Part model, mm, in its own coordinate system. A direction names the side the tool comes from. Round coordinates to 2 decimals unless told otherwise and drop trailing zeros. Write each loop counter-clockwise with the first axis right and the second up, starting at its lowest first coordinate (ties: lowest second). Pieces come first, ordered by that corner, then holes.
```python
from build123d import *

# Parameters (mm, degrees)
CHAMFER_1_SIZE           = 1
CHAMFER_2_SIZE           = 1
CHAMFER_3_SIZE           = 1
FILLET_1_R               = 2
SKETCH_2_R               = 4.5
CUT_EXTRUDE_1_DEPTH      = 72.003521039
CUT_EXTRUDE_START        = -13
SKETCH_3_R               = 7
CUT_EXTRUDE_2_DEPTH      = 9
PATTERN_CIRCULAR_2_COUNT = 4


with BuildPart() as part:
    # 草图1 → 旋转1 (revolve)
    with BuildSketch(Plane.XY, mode=Mode.PRIVATE) as revolve_1_sk:
        Polygon((45, 11), (45, 17), (23, 27.5), (23, 47.5), (10, 47.5), (10, 31), (0, 31), (0, 22.5), (15, 22.5), (15, 11), align=None)
    revolve(revolve_1_sk.sketch.rotate(Axis((0, 0, 0), (1, 0, 0)), 90), axis=Axis((0, 0, 0), (1, 0, 0)))

    # 倒角1
    chamfer_1_edges = [part.edges().sort_by_distance(p)[0] for p in [
        (45, 0, -11),
    ]]
    chamfer(chamfer_1_edges, length=CHAMFER_1_SIZE)

    # 倒角2
    chamfer_2_edges = [part.edges().sort_by_distance(p)[0] for p in [
        (0, 0, -31),
    ]]
    chamfer(chamfer_2_edges, length=CHAMFER_2_SIZE)

    # 倒角3
    chamfer_3_edges = [part.edges().sort_by_distance(p)[0] for p in [
        (23, 0, -47.5),
    ]]
    chamfer(chamfer_3_edges, length=CHAMFER_3_SIZE)

    # 圆角1
    fillet_1_edges = [part.edges().sort_by_distance(p)[0] for p in [
        (23, 0, -27.5),
    ]]
    fillet(fillet_1_edges, radius=FILLET_1_R)

    # 草图2 → 切除-拉伸1 (cut, through all)
    with BuildSketch(Plane(origin=(23, 0, 0), x_dir=(0, 0, -1), z_dir=(1, 0, 0))):
        with Locations((0, 39)):
            Circle(SKETCH_2_R)
    cut_extrude_1 = extrude(amount=-CUT_EXTRUDE_1_DEPTH, mode=Mode.SUBTRACT)

    # 草图3 → 切除-拉伸2 (cut)
    with BuildSketch(Plane.ZY.offset(-10).offset(CUT_EXTRUDE_START)):
        with Locations((0, 39)):
            Circle(SKETCH_3_R)
    cut_extrude_2 = extrude(amount=CUT_EXTRUDE_2_DEPTH, mode=Mode.SUBTRACT)

    # 阵列(圆周)2: 切除-拉伸1, 切除-拉伸2 ×4 about axis
    pattern_circular_2_axis = Axis((0, 0, 0), (1, 0, 0))
    add([cut_extrude_1.rotate(pattern_circular_2_axis, i * 360 / PATTERN_CIRCULAR_2_COUNT) for i in range(1, PATTERN_CIRCULAR_2_COUNT)], mode=Mode.SUBTRACT)
    add([cut_extrude_2.rotate(pattern_circular_2_axis, i * 360 / PATTERN_CIRCULAR_2_COUNT) for i in range(1, PATTERN_CIRCULAR_2_COUNT)], mode=Mode.SUBTRACT)


solid = part.part
```
Q1. Cut at C-C on x = 38.5. Write the cut outline in (y, z), plus the area to 3 significant figures.
Values follow:
outline: circle Ø40.2 at (0, 0); hole circle Ø22 at (0, 0)
area: 889 mm2
Q2. Wall check: L1, parallel to Y at x = 16.25, z = 0; L2, parallel to Y at x = 12, z = 0; L3, parallel to Z at x = 20, y = -5.5. Give the ranges that are in metal, low to high.
Values follow:
L1: y = -47.5 to -46, -32 to -11, 11 to 32, 46 to 47.5
L2: y = -47.5 to -43.5, -34.5 to -22.5, 22.5 to 34.5, 43.5 to 47.5
L3: z = -47.18 to -43.33, -34.67 to -9.53, 9.53 to 34.67, 43.33 to 47.18
Q3. Cut at A-A on x = 12.5. Write the cut outline in (y, z).
Values follow:
outline: circle Ø95 at (0, 0); hole circle Ø9 at (-39, 0); hole circle Ø45 at (0, 0); hole circle Ø9 at (0, -39); hole circle Ø9 at (0, 39); hole circle Ø9 at (39, 0)
Q4. Mould opens along Z. For faces 1 (the flat face through (14, 5, -39)), 2 (the cylindrical face through (5.437, -30.736, -4.036)), 3 (the flat face through (0, -22.4, 4.3)) say: +Z half, -Z half, draft (parallel to the pull), parting line (faces both ways), or undercut.
Values follow:
face 1: undercut
face 2: parting line
face 3: draft
Q5. Cut at B-B on z = 0. State how many separate pieces and enclosed holes the cut face has, plus the area to 3 significant figures.
Values follow:
separate pieces: 4
enclosed holes: 0
area: 1,170 mm2
Q6. Drop flat-ended pins along their axis: pin 1 (8 mm diameter, centred on x = 40, z = -6.5, fed in from +Y); pin 2 (10 mm diameter, centred on x = 7, z = -8.5, fed in from -Y); pin 3 (11.5 mm diameter, centred on y = -39, z = 0, fed in from +X). Give the stop position or say it passes through.
Values follow:
pin 1: stops at y = 20.56
pin 2: stops at y = -47.29
pin 3: stops at x = 14
Q7. Cut at D-D on x = 3. Write the cut outline in (y, z), plus the area to 3 significant figures.
Values follow:
outline: circle Ø62 at (0, 0); hole circle Ø45 at (0, 0)
area: 1,430 mm2
Q8. Which spindle directions (+Z, -Z, +X, -X, +Y, -Y) get a long thin tool onto all of the face, cutting with end or side? Do faces 4 (the cylindrical face through (29.7, 10.74, -2.38)), 5 (the cylindrical face through (18.56, -0.91, -45.94)), 6 (the cylindrical face through (7.605, 19.961, 10.382)). Say none if no direction does.
Values follow:
face 4: +X, -X
face 5: +X
face 6: -X
